Geometry: final body of the model. Coordinates: model frame, mm. Round coordinates to 2 decimals unless told otherwise and drop trailing zeros. Loops run counter-clockwise (first coordinate to the right, second up) from the corner with the lowest first, then second, coordinate; pieces in that order, holes last. Notation, with made-up numbers: M 47.25,4.25 L 88.25,4.25 A21 cw 88.25,41.25 Z; hole C 86.5,20.25 d11. An arc over 180 degrees is marked long. Write each question's results on one line, items separated by ' | '.
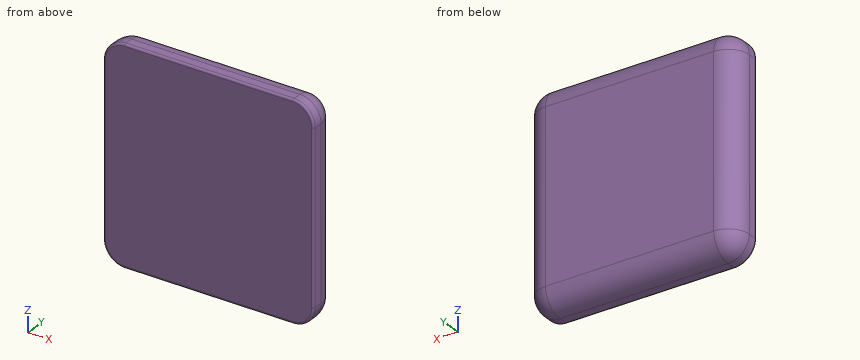
```python
from build123d import *

# Parameters (mm, degrees)
F0_W     = 254
F0_H     = 254
F1_DEPTH = 38.1
F2_R     = 25.4
F3_R     = 25.4
F4_R     = 25.4
F5_R     = 25.4
F6_R     = 2.54
F7_R     = 25.4


with BuildPart() as f1:
    # F0 (on Front) → F1 (new body)
    with BuildSketch(Plane.XZ):
        with Locations((127, 127)):
            Rectangle(F0_W, F0_H)
    extrude(amount=F1_DEPTH)

    # F2
    f2_edges = [f1.edges().sort_by_distance(p)[0] for p in [
        (0, -19.05, 254),
    ]]
    fillet(f2_edges, radius=F2_R)

    # F3
    f3_edges = [f1.edges().sort_by_distance(p)[0] for p in [
        (0, -19.05, 0),
    ]]
    fillet(f3_edges, radius=F3_R)

    # F4
    f4_edges = [f1.edges().sort_by_distance(p)[0] for p in [
        (254, -19.05, 0),
    ]]
    fillet(f4_edges, radius=F4_R)

    # F5
    f5_edges = [f1.edges().sort_by_distance(p)[0] for p in [
        (254, -19.05, 254),
    ]]
    fillet(f5_edges, radius=F5_R)

    # F6
    f6_edges = [f1.edges().sort_by_distance(p)[0] for p in [
        (254, -38.1, 127),
    ]]
    fillet(f6_edges, radius=F6_R)

    # F7
    f7_edges = [f1.edges().sort_by_distance(p)[0] for p in [
        (254, 0, 127),
    ]]
    fillet(f7_edges, radius=F7_R)


solid = f1.part
```
1. Section A-A (x = 71). Output: boundary loops of the cut face in (y, z).
Answer key:
outline: M -38.1,2.54 A2.54 ccw -35.56,0 L -25.4,0 A25.4 ccw 0,25.4 L 0,228.6 A25.4 ccw -25.4,254 L -35.56,254 A2.54 ccw -38.1,251.46 Z
2. Ray query, probe 1 along X at (y, z) = (-36, 117.5); probe 2 along Z at (x, y) = (224, -25); probe 3 along Z at (x, y) = (116, -22.5). Return the intervals inside material, ascending.
Answer key:
probe 1: x = 0.04 to 253.96 | probe 2: z = 0 to 254 | probe 3: z = 0.17 to 253.83
3. Section B-B (y = -7). Output: boundary loops of the cut face in (x, z), then the cut area to 3 significant figures.
Answer key:
outline: M 7.89,25.4 A17.51 ccw 25.4,7.89 L 228.6,7.89 A17.51 ccw 246.11,25.4 L 246.11,228.6 A17.51 ccw 228.6,246.11 L 25.4,246.11 A17.51 ccw 7.89,228.6 Z | area: 56,500 mm²
4. Pin query (flat end, axial travel): P1, Ø2, axis at y = -5.5, z = 156.5, coming from the -X side; P2, Ø4, axis at x = 203.5, y = -6.5, coming from the +Z side; P3, Ø10, axis at x = 137, y = -18, coming from the +Z side. Return the tip coordinate at first contact, or that it passes through.
Answer key:
P1: stops at x = 8.43 | P2: stops at z = 247.56 | P3: stops at z = 253.89
